```python
from build123d import *

# Parameters (mm, degrees)
FILLET1_R   = 0.25
HEX_START   = -2.2
HEX_2_DEPTH = 2.2


with BuildPart() as part:
    # BodySke → BaseBody (revolve)
    with BuildSketch(Plane.XY, mode=Mode.PRIVATE) as basebody_sk:
        Polygon((0, 0), (0, 5.85), (0.87, 5.85), (3.72, 3), (11.4455, 3), (12, 2.4455), (12, 0), align=None)
    revolve(basebody_sk.sketch.rotate(Axis((0, 0, 0), (1, 0, 0)), 90), axis=Axis((0, 0, 0), (1, 0, 0)))

    # Fillet1
    fillet1_edges = [part.edges().sort_by_distance(p)[0] for p in [
        (3.72, 0, -3),
    ]]
    fillet(fillet1_edges, radius=FILLET1_R)

    # Hex 2: read off the stored shape, not the designer's step
    # Hex 2 outline → Hex 2 (cut)
    with BuildSketch(Plane.ZY.offset(HEX_START)):
        Polygon((-2, -1.154700538), (0, -2.309401077), (2, -1.154700538), (2, 1.154700538), (0, 2.309401077), (-2, 1.154700538), align=None)
    extrude(amount=HEX_2_DEPTH, mode=Mode.SUBTRACT)

    # Hex 2 2 outline → Hex 2 2 (revolve, cut)
    with BuildSketch(Plane.YX):
        Polygon((2, 2.2), (0, 3.354700538), (0, 2.2), align=None)
    revolve(axis=Axis((0, 0, 0), (1, 0, 0)), mode=Mode.SUBTRACT)


solid = part.part
```
Geometry check sheet. Reference: the model listing, model coordinates, mm. A direction names the side the tool comes from. Coordinates: 2 decimals unless noted, no trailing zeros. Order: outer loops, then holes, each group sorted by start corner. A loop starts at its lowest first (then second) coordinate and runs counter-clockwise, first axis right, second up. Notation, with made-up numbers: M 37.25,3.5 L 43.25,3.5 A25 cw 43.25,37.5 Z; hole C 21.5,-7.75 d6. An arc over 180 degrees is marked long. One line per question, with ' | ' between items. Start each with the question number.
Item 1: Gauge pin test, flat ends, axial feed: pin 1 (6 mm diameter, centred on x = 6, y = -2, fed in from +Z); pin 2 (3 mm diameter, centred on y = -4, z = -4.5, fed in from -X); pin 3 (3 mm diameter, centred on x = 3, z = 2.5, fed in from -Y); pin 4 (1 mm diameter, centred on x = 10.5, z = 1.5, fed in from -Y). Record the tip position at first contact, or that the pin passes through.
Item 2: Material ranges on L1, parallel to X at y = -1.25, z = -1.75; L2, parallel to Y at x = 7.75, z = 0; L3, parallel to Y at x = 1.75, z = -3, recorded low to high. Write a range as [from, to].
Item 3: Draft check along Y on faces 1 (the flat face through (0, 0, -3)), 2 (the flat face through (1.115, 1.724, 1.014)), 3 (the conical face through (3.512, -0.964, 3.06)). Enter one of: pulls with the +Y half, pulls with the -Y half, needs draft (parallel to the pull), parting line crosses it, or undercut.
Item 4: Set-up check for faces 4 (the flat face through (1.12, -1.74, 0.99)), 5 (the flat face through (12, 0, 0)), 6 (the cylindrical face through (7.69, -0.9, 2.86)): record each of +Z, -Z, +X, -X, +Y, -Y from which the full face is reachable in a straight line by a thin tool's end or side.
Item 5: Cross-section at A-A on x = 10.25. Enter the section's corners in (y, z).
Findings:
1) pin 1: stops at z = 3.41 | pin 2: stops at x = 0 | pin 3: stops at y = -4.73 | pin 4: stops at y = -2.83
2) L1: x = [2.2, 12] | L2: y = [-3, 3] | L3: y = [-3.96, 3.96]
3) face 1: needs draft | face 2: undercut | face 3: parting line crosses it
4) face 4: -X | face 5: +Z, -Z, +X, +Y, -Y | face 6: +X
5) outline: C 0,0 d6
